Here's how the part is built. I have some questions about the finished solid (model axes, mm). Coordinates: 2 decimals unless noted, no trailing zeros. Loops run counter-clockwise (first coordinate to the right, second up) from the corner with the lowest first, then second, coordinate; pieces in that order, holes last. Notation, with made-up numbers: (15, -17.75) - (68, -17.75) arc R36 ccw to (68, 18.25) - close; hole circle Ø1 at (86, -24.5). An arc over 180 degrees is marked (long way). Use a Markdown table: item, result.
Solid Edge part; units mm, degrees
sketch "Sketch1" plane through (0, 0, 0) normal (0, 0, 1) x (1, 0, 0)
  line L0 (8.2849, 4.8418) -> (98.2849, 4.8418)
  line L1 (98.2849, 4.8418) -> (98.2849, 20.8418)
  line L2 (8.2849, 124.8418) -> (98.2849, 20.8418)
  line L3 (8.2849, 4.8418) -> (8.2849, 124.8418)
extrude "Protrusion1" add sketch "Sketch1" along normal blind 12
sketch "Sketch2" plane through (53.2849, 64.8418, 12) normal (0, 0, 1) x (1, 0, 0)
  line L0 (-45, -48.7017) -> (-33.6863, -60.0155)
  line L1 (-33.6863, -60.0155) -> (-45, -60)
  line L2 (-45, -60) -> (-45, -48.7017)
  line L3 (-45, 45.8836) -> (-32.7839, 45.8836)
  line L4 (-32.7839, 45.8836) -> (-45, 60)
  line L5 (-45, 60) -> (-45, 45.8836)
extrude "ExtrudedCutout_1" cut sketch "Sketch2" against normal blind 382.4584
Q1. Please list where these lines run through material, in increasing order: L1, parallel to X at y = 72, z = 10.25; L2, parallel to Y at x = 28, z = 5.5; L3, parallel to Y at x = 67, z = 10.25. Write a range as from..to.
Check values:
| item | result |
|---|---|
| L1 | 8.28..54.01 |
| L2 | 4.84..102.06 |
| L3 | 4.84..56.99 |
Q2. I want a section at A-A, the plane z = 10. Write out the boundary of the cut face in (x, y).
Check values:
| item | result |
|---|---|
| outline | (8.28, 16.14) - (19.58, 4.84) - (98.28, 4.84) - (98.28, 20.84) - (20.5, 110.73) - (8.28, 110.73) - close |
Q3. I want a section at C-C, the plane x = 48. Write out the boundary of the cut face in (y, z).
Check values:
| item | result |
|---|---|
| outline | (4.84, 0) - (78.95, 0) - (78.95, 12) - (4.84, 12) - close |
Q4. Will these pins go through, and if not, where does the flat tip stop? P1, Ø6, axis at x = 23, y = 47, coming from the -Z side; P2, Ø1, axis at x = 64.5, z = 7.5, coming from the +Y side; P3, Ø6, axis at x = 61, z = 10, coming from the +Y side; P4, Ø5, axis at y = 30.5, z = 7, coming from the +X side.
Check values:
| item | result |
|---|---|
| P1 | z = 0 |
| P2 | y = 60.46 |
| P3 | y = 67.39 |
| P4 | x = 92.09 |
Q5. I want a section at B-B, the plane y = 22.5. Write out the boundary of the cut face in (x, z), then the cut area to 3 significant figures.
Check values:
| item | result |
|---|---|
| outline | (8.28, 0) - (96.85, 0) - (96.85, 12) - (8.28, 12) - close |
| area | 1,060 mm^2 |
